from build123d import *

# Parameters (mm, degrees)
F1_DEPTH = 25.4


with BuildPart() as f1:
    # F0 (on Top) → F1 (new body)
    with BuildSketch(Plane.XY):
        Polygon((15.0094395503, 0), (0, 0), (0, -41.2759594619), (49.8700737953, -41.2759594619), (49.8700737953, -20.637979731), (15.0094395503, -20.637979731), align=None)
    extrude(amount=F1_DEPTH)

    # F2: sweep along a path in F2_path
    with BuildLine(Plane(origin=(49.8700737953, -41.2759594619, 25.4), x_dir=(0, 0, 1), z_dir=(0, -1, 0))) as f2_path:
        Line((0, 0), (-25.4, 0))
    # F1_face (on face) → F2 (sweep)
    with BuildSketch(Plane(origin=(20.9026501287, -26.1825116321, 25.4), x_dir=(1, 0, 0), z_dir=(0, 0, 1))):
        Polygon((-5.8932105783, 26.1825116321), (-20.9026501287, 26.1825116321), (-20.9026501287, -15.0934478298), (28.9674236666, -15.0934478298), (28.9674236666, 5.5445319012), (-5.8932105783, 5.5445319012), align=None)
    sweep(path=f2_path.line)


solid = f1.part
Geometry check sheet. Reference: the model listing, model coordinates, mm. A direction names the side the tool comes from. Coordinates: 2 decimals unless noted, no trailing zeros. Order: outer loops, then holes, each group sorted by start corner. A loop starts at its lowest first (then second) coordinate and runs counter-clockwise, first axis right, second up. Notation, with made-up numbers: (-6.75, 49) - (29.25, 49) arc R34 ccw to (29.25, 83) - close; hole circle Ø3 at (13.25, 77.25). An arc over 180 degrees is marked (long way). One line per item, written item: value.
(1) Thickness scan on probe 1 along X at (y, z) = (-9.5, 2.75); probe 2 along Y at (x, z) = (29.5, 2). Record the ranges inside material, lowest first. Write a range as from..to.
Data:
probe 1: x = 0..15.01
probe 2: y = -41.28..-20.64
(2) Sectioned sample at B-B (y = -20). Enter the section's corners in (x, z), and give its area (3 significant figures).
Data:
outline: (0, 0) - (15.01, 0) - (15.01, 25.4) - (0, 25.4) - close
area: 381 mm^2
(3) Sectioned sample at A-A (z = 14.75). Enter the section's corners in (x, y), and give its area (3 significant figures).
Data:
outline: (0, -41.28) - (49.87, -41.28) - (49.87, -20.64) - (15.01, -20.64) - (15.01, 0) - (0, 0) - close
area: 1,340 mm^2
(4) Sectioned sample at C-C (x = 38.5). Enter the section's corners in (y, z).
Data:
outline: (-41.28, 0) - (-20.64, 0) - (-20.64, 25.4) - (-41.28, 25.4) - close
(5) Depth check by flat-ended pin: pin 1 Ø1.5 at (x, z) = (35.5, 18.5) entering from +Y; pin 2 Ø1 at (y, z) = (-20, 5.5) entering from +X. Enter the tip coordinate at first touch or a pass-through.
Data:
pin 1: stops at y = -20.64
pin 2: stops at x = 15.01
(6) Access from +Z, -Z, +X, -X, +Y, -Y to the whole of each face (thin tool, end or side, straight path). Record for faces 1 (the face through (33, -20.638, 13)), 2 (the face through (19, -25, 0)).
Data:
face 1: +Z, -Z, +X, +Y
face 2: -Z, +X, -X, +Y, -Y
